Build history of the part. All positions in model axes, mm. A direction names the side the tool comes from. Give positions to 0.01 mm unless a question says otherwise; leave off trailing zeros. Write each loop counter-clockwise with the first axis right and the second up, starting at its lowest first coordinate (ties: lowest second). Pieces come first, ordered by that corner, then holes. Notation, with made-up numbers: (76.25, -6.75) -> (125.25, -6.75) arc R13 cw to (125.25, 15.25) -> close; hole circle Ø9 at (44.25, -4). An arc over 180 degrees is marked (long way). Put each result on its own line as item: value. Start each with the question number.
Item 1: Tool access for faces 5 (the cylindrical face through (15.5, 4.88, 6.51)), 6 (the cylindrical face through (-22.12, -25.33, 0.11)), 7 (the flat face through (-20.944, -19.285, 0.105)), 8 (the flat face through (15.5, -16, 0)), 9 (the flat face through (-16.23, -23.465, 0.105)): list every direction of +Z, -Z, +X, -X, +Y, -Y with a clear straight run to the whole face (end or side of a thin tool).
Item 2: Two-plate mould, pull along X, no slides. Class faces 1 (the cylindrical face through (-7.124, -24.485, 0.105)), 2 (the flat face through (25.5, -16, -7)), 3 (the flat face through (21, -7.1, 0)), 4 (the flat face through (0, 0, 5.5)): pulls with the +X half, pulls with the -X half, needs draft (parallel to the pull), parting line crosses it, or undercut.
Item 3: Flat gauge pins, fed straight in: pin 1 Ø5 at (y, z) = (2, -1.5) entering from -X; pin 2 Ø10 at (x, y) = (-3, -3) entering from +Z; pin 3 Ø1 at (x, z) = (18.5, -4.5) entering from -Y; pin 4 Ø12 at (x, y) = (5, -15) entering from +Z. Where does each tip first touch, or does it go through?
Item 4: Slice it at C-C, the plane z = -3. List the corners of the cut face in (x, y), plus the area to 3 significant figures.
Item 5: Drill centre lines: line 1 along Y through (x, z) = (18, 3); line 2 along Y through (x, z) = (0, 6.1); line 3 along Z through (x, y) = (9, 11). Where is each one in solid material? Low to high.
Item 6: Slice it at A-A, the plane y = -23. List the corners of the cut face in (x, z), plus the area to 3 significant figures.
Item 7: Slice it at D-D, the plane x = -7. List the corners of the cut face in (y, z) (3 decimals), plus the area to 3 significant figures.
Item 8: Slice it at B-B, the plane y = 20.5. List the corners of the cut face in (x, z), plus the area to 3 significant figures.
```python
from build123d import *

# Parameters (mm, degrees)
SKETCH1_R           = 3.15
SKETCH1_R_2         = 2.15
BOSS_EXTRUDE1_DEPTH = 7.5
SKETCH3_W           = 2
SKETCH3_H           = 0.9
BOSS_EXTRUDE2_DEPTH = 11.4
SKETCH4_R           = 16.25
CUT_EXTRUDE1_DEPTH  = 2
SKETCH5_W           = 12.5
SKETCH5_H           = 17.5
CUT_EXTRUDE2_DEPTH  = 10


with BuildPart() as part:
    # Sketch1 → Boss-Extrude1 (new, symmetric)
    # profile 1 of 5: a face of its own
    with BuildSketch(Plane.XY):
        with BuildLine():
            ThreePointArc((-13.512663894, -21.625399753), (-7.028595389, -24.512218318), (0, -25.5))
            Line((0, -25.5), (0, -6.2))
            Line((0, -6.2), (22.3, -6.2))
            ThreePointArc((22.3, -6.2), (22.633696889, 4.842082728), (17.811452389, 14.781142168))
            ThreePointArc((17.811452389, 14.781142168), (17.583444291, 15.489857701), (17.908337826, 16.159715588))
            Line((17.908337826, 16.159715588), (18.928412767, 17.086988913))
            Line((18.928412767, 17.086988913), (20.118834813, 18.169111965))
            ThreePointArc((20.118834813, 18.169111965), (15.669111965, 18.381165187), (15.881165187, 22.830888035))
            Line((15.881165187, 22.830888035), (14.69074314, 21.748764984))
            ThreePointArc((14.69074314, 21.748764984), (14.108162444, 21.492793575), (13.489112369, 21.64009814))
            ThreePointArc((13.489112369, 21.64009814), (-19.251546311, 16.722080152), (-19.539541583, -16.384636545))
            ThreePointArc((-19.539541583, -16.384636545), (-19.305838355, -17.036142145), (-19.551192594, -17.683350027))
            Line((-19.551192594, -17.683350027), (-22.377007395, -20.933037048))
            ThreePointArc((-22.377007395, -20.933037048), (-18.896612782, -20.049570091), (-16.85, -23))
            ThreePointArc((-16.85, -23), (-17.049570091, -24.103387218), (-17.622992605, -25.066962952))
            Line((-17.622992605, -25.066962952), (-14.797177804, -21.817275931))
            ThreePointArc((-14.797177804, -21.817275931), (-14.190309608, -21.484428012), (-13.512663894, -21.625399753))
        make_face()
    # profile 2 of 5: a face of its own
    with BuildSketch(Plane.XY):
        with Locations((-20, -23)):
            Circle(SKETCH1_R)
        with Locations((-20, -23)):
            Circle(SKETCH1_R_2, mode=Mode.SUBTRACT)
    # profile 3 of 5: a face of its own
    with BuildSketch(Plane.XY):
        with Locations((18, 20.5)):
            Circle(SKETCH1_R)
        with Locations((18, 20.5)):
            Circle(SKETCH1_R_2, mode=Mode.SUBTRACT)
    # profile 4 of 5: a face of its own
    with BuildSketch(Plane.XY):
        with BuildLine():
            Line((0, -6.2), (0, -25.5))
            ThreePointArc((0, -25.5), (15.686777872, -20.104104059), (24.734793308, -6.2))
            Line((24.734793308, -6.2), (22.3, -6.2))
            Line((22.3, -6.2), (0, -6.2))
        make_face()
    # profile 5 of 5: a face of its own
    with BuildSketch(Plane.XY):
        with BuildLine():
            Line((0, -25.5), (25.5, -25.5))
            Line((25.5, -25.5), (25.5, -6.2))
            Line((25.5, -6.2), (24.734793308, -6.2))
            ThreePointArc((24.734793308, -6.2), (15.686777872, -20.104104059), (0, -25.5))
        make_face()
    extrude(amount=BOSS_EXTRUDE1_DEPTH, both=True)

    # Sketch3 → Boss-Extrude2 (add)
    with BuildSketch(Plane(origin=(25.5, 0, 0), x_dir=(0, 0, -1), z_dir=(1, 0, 0))):
        with Locations((0.3, -25.95)):
            Rectangle(SKETCH3_W, SKETCH3_H)
    extrude(amount=-BOSS_EXTRUDE2_DEPTH)

    # Sketch4 → Cut-Extrude1 (cut)
    with BuildSketch(Plane.XY.offset(7.5)):
        Circle(SKETCH4_R)
    extrude(amount=-CUT_EXTRUDE1_DEPTH, mode=Mode.SUBTRACT)

    # Sketch5 → Cut-Extrude2 (cut)
    with BuildSketch(Plane(origin=(25.5, 0, 0), x_dir=(0, 0, -1), z_dir=(1, 0, 0))):
        with Locations((0, -15.85)):
            Rectangle(SKETCH5_W, SKETCH5_H)
    extrude(amount=-CUT_EXTRUDE2_DEPTH, mode=Mode.SUBTRACT)


solid = part.part
```
Values follow:
1. face 5: +Z
1. face 6: +Z, -Z
1. face 7: +Z, -Z, -X
1. face 8: +X
1. face 9: +Z, -Z, -Y
2. face 1: undercut
2. face 2: pulls with the +X half
2. face 3: needs draft
2. face 4: undercut
3. pin 1: x = -25.5
3. pin 2: z = 5.5
3. pin 3: y = -25.5
3. pin 4: z = 7.5
4. outline: (-22.38, -20.93) arc R3.15 ccw to (-17.62, -25.07) -> (-14.8, -21.82) arc R1 cw to (-13.51, -21.63) arc R25.5 ccw to (0, -25.5) -> (25.5, -25.5) -> (25.5, -24.6) -> (15.5, -24.6) -> (15.5, -7.1) -> (25.5, -7.1) -> (25.5, -6.2) -> (22.3, -6.2) arc R23.15 ccw to (17.81, 14.78) arc R1 cw to (17.91, 16.16) -> (20.12, 18.17) arc R3.15 ccw to (15.88, 22.83) -> (14.69, 21.75) arc R1 cw to (13.49, 21.64) arc R25.5 ccw to (-19.54, -16.38) arc R1 cw to (-19.55, -17.68) -> close; hole circle Ø4.3 at (-20, -23); hole circle Ø4.3 at (18, 20.5)
4. area: 2,000 mm2
5. line 1: -25.5 to -24.6, -7.1 to 14.55, 16.24 to 18.35, 22.65 to 23.65
5. line 2: -25.5 to -16.25, 16.25 to 25.5
5. line 3: -7.5 to 5.5
6. outline: (-23.15, -7.5) -> (-22.15, -7.5) -> (-22.15, 7.5) -> (-23.15, 7.5) -> close; (-17.85, -7.5) -> (-15.83, -7.5) -> (-15.83, 7.5) -> (-17.85, 7.5) -> close; (-11.01, -7.5) -> (25.5, -7.5) -> (25.5, -6.25) -> (15.5, -6.25) -> (15.5, 6.25) -> (25.5, 6.25) -> (25.5, 7.5) -> (-11.01, 7.5) -> close
6. area: 468 mm2
7. outline: (-24.52, -7.5) -> (24.52, -7.5) -> (24.52, 7.5) -> (14.665, 7.5) -> (14.665, 5.5) -> (-14.665, 5.5) -> (-14.665, 7.5) -> (-24.52, 7.5) -> close
7. area: 677 mm2
8. outline: (-15.17, -7.5) -> (15.85, -7.5) -> (15.85, 7.5) -> (-15.17, 7.5) -> close; (20.15, -7.5) -> (21.15, -7.5) -> (21.15, 7.5) -> (20.15, 7.5) -> close
8. area: 480 mm2
